The figure shows three views and two pictorial views of one solid part (mm, origin at its lowest corner). Answer the questions. A direction names the side the tool comes from. Round coordinates to 2 decimals unless told otherwise and drop trailing zeros. Order: outer loops, then holes, each group sorted by start corner. A loop starts at its lowest first (then second) coordinate and runs counter-clockwise, first axis right, second up. Notation, with made-up numbers: (7, 50) -> (52, 50) arc R21 cw to (52, 66) -> close; hole circle Ø7 at (-2, 22.5). An arc over 180 degrees is marked (long way). Answer in a Markdown table with one row per item. Add a question column.
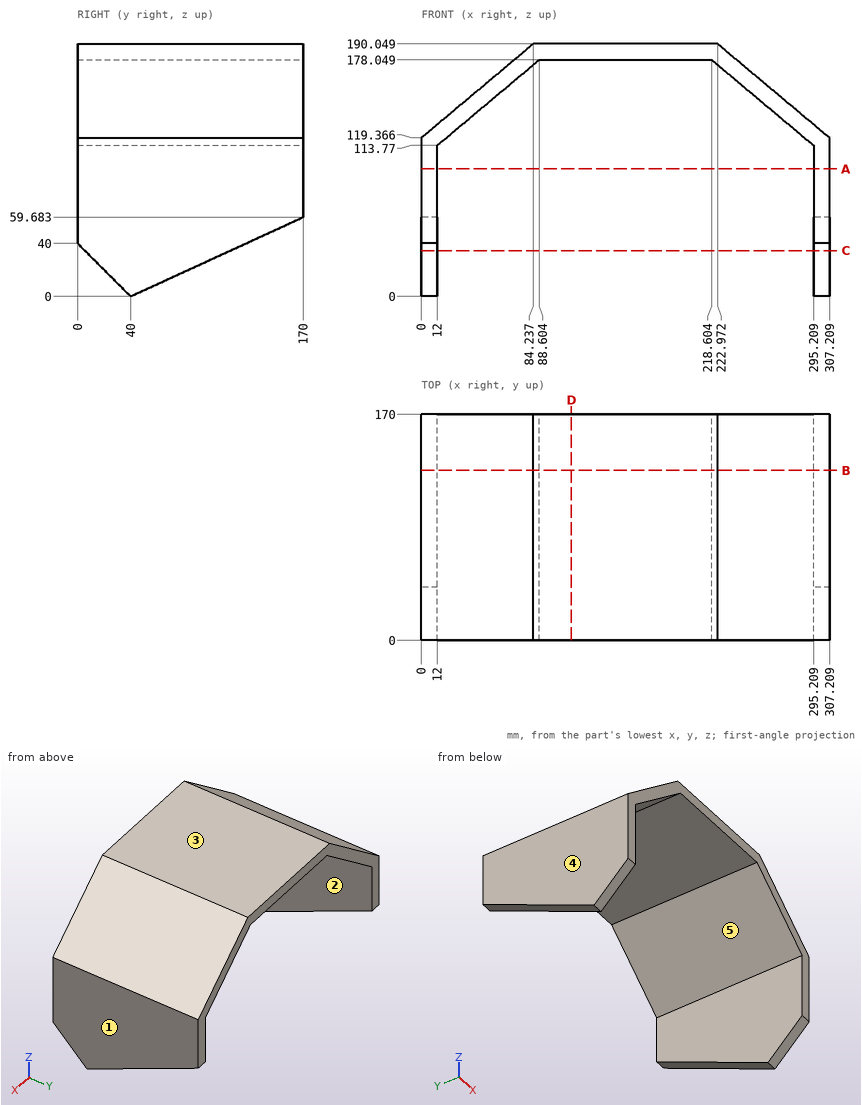
1. For the marked faces 1 and 2, determine the directions among +Z, -Z, +X, -X, +Y, -Y from which every point of the face is accessible in a straight line to the end or side of a thin tool.
2. The part is cut by section C-C (z = 34.5). Give the vertices of the cut face in (x, y), then the cut area to 3 significant figures.
3. The part is cut by section A-A (z = 96). Give the vertices of the cut face in (x, y).
4. Each of these flat-tipped pins is pushed along its axis until it touches: pin 1 (1.5 mm diameter, centred on y = 75.5, z = 146.5, fed in from +X) (1 decimal); pin 2 (4 mm diameter, centred on y = 20.5, z = 139, fed in from +X) (1 decimal). Where does it stop, or does it pass through?
5. The part is cut by section B-B (y = 128). Give the vertices of the cut face in (x, z) (1 decimal), then the cut area to 3 significant figures.
6. The part is cut by section D-D (x = 113). Give the vertices of the cut face in (y, z).
7. Straight lines are drawn through the part: line 1 along X through (y, z) = (119.5, 77.5); line 2 along Z through (x, y) = (196, 48); line 3 along X through (y, z) = (75.5, 114) (1 decimal). For each, find the intervals that lie inside material, in ascending order.
8. The mould has two halves that part along X. Classify the marked faces 3, 4 and 5: released by +X, released by -X, zero draft, split by the parting line, or undercut.
Report:
| question | item | result |
|---|---|---|
| 1 | face 1 | +Z, -Z, +X, +Y, -Y |
| 1 | face 2 | -Z, +Y, -Y |
| 2 | outline | (0, 5.5) -> (12, 5.5) -> (12, 115.15) -> (0, 115.15) -> close; (295.21, 5.5) -> (307.21, 5.5) -> (307.21, 115.15) -> (295.21, 115.15) -> close |
| 2 | area | 2,630 mm^2 |
| 3 | outline | (0, 0) -> (12, 0) -> (12, 170) -> (0, 170) -> close; (295.21, 0) -> (307.21, 0) -> (307.21, 170) -> (295.21, 170) -> close |
| 4 | pin 1 | stops at x = 275.8 |
| 4 | pin 2 | stops at x = 286.2 |
| 5 | outline | (0, 40.4) -> (12, 40.4) -> (12, 113.8) -> (88.6, 178) -> (218.6, 178) -> (295.2, 113.8) -> (295.2, 40.4) -> (307.2, 40.4) -> (307.2, 119.4) -> (223, 190) -> (84.2, 190) -> (0, 119.4) -> close |
| 5 | area | 5,960 mm^2 |
| 6 | outline | (0, 178.05) -> (170, 178.05) -> (170, 190.05) -> (0, 190.05) -> close |
| 7 | line 1 | x = 0 to 12, 295.21 to 307.21 |
| 7 | line 2 | z = 178.05 to 190.05 |
| 7 | line 3 | x = 0 to 12.3, 294.9 to 307.2 |
| 8 | face 3 | zero draft |
| 8 | face 4 | released by -X |
| 8 | face 5 | undercut |
